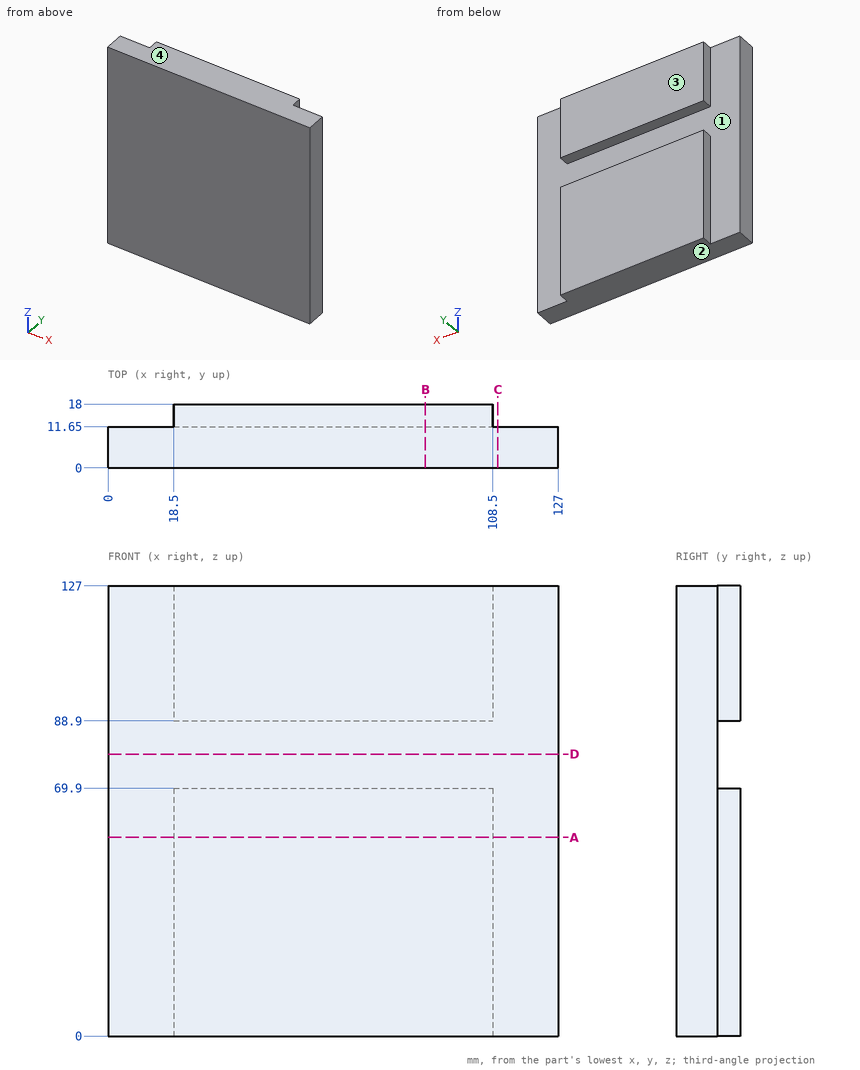
For this review, use the dimensioned drawing (mm, ordinates from the lowest corner) and the shaded views. Coordinates: 2 decimals unless noted, no trailing zeros. Loops run counter-clockwise (first coordinate to the right, second up) from the corner with the lowest first, then second, coordinate; pieces in that order, holes last. Notation, with made-up numbers: (9.25, -37) -> (47.25, -37) arc R27 cw to (47.25, -3) -> close; hole circle Ø1 at (52.5, 73). An arc over 180 degrees is marked (long way). Write each question's results on one line, items separated by ' | '.
Q1. Add section D-D, the plane z = 79.5. State the section outline as (x, y) points.
Taken from the geometry:
outline: (0, 0) -> (127, 0) -> (127, 11.65) -> (0, 11.65) -> close
Q2. To check wall thickness, follow line 1 along Z through (x, y) = (35.5, 14.25); line 2 along X through (y, z) = (12, 43.5); line 3 along Y through (x, z) = (26.5, 78). State the ranges of each line that lie inside material, in increasing order. Write a range as [from, to].
Taken from the geometry:
line 1: [0, 69.9], [88.9, 127] | line 2: [18.5, 108.5] | line 3: [0, 11.65]
Q3. Add section A-A, the plane z = 56. State the section outline as (x, y) points.
Taken from the geometry:
outline: (0, 0) -> (127, 0) -> (127, 11.65) -> (108.5, 11.65) -> (108.5, 18) -> (18.5, 18) -> (18.5, 11.65) -> (0, 11.65) -> close
Q4. Add section C-C, the plane x = 110. State the section outline as (y, z) points, then the cut area to 3 significant figures.
Taken from the geometry:
outline: (0, 0) -> (11.65, 0) -> (11.65, 127) -> (0, 127) -> close | area: 1,480 mm²
Q5. For pin 1 Ø3 at (y, z) = (14.5, 106) entering from +X; pin 2 Ø7 at (y, z) = (15.5, 45.5) entering from -X, all flat-tipped, find the tip position at first contact; note any pin that passes through.
Taken from the geometry:
pin 1: x = 108.5 | pin 2: x = 18.5
Q6. Add section B-B, the plane x = 89.5. State the section outline as (y, z) points.
Taken from the geometry:
outline: (0, 0) -> (18, 0) -> (18, 69.9) -> (11.65, 69.9) -> (11.65, 88.9) -> (18, 88.9) -> (18, 127) -> (0, 127) -> close
Q7. Mouldability with a two-part tool opening along Z and no side actions: class the marked faces 1, 2, 3 and 4 as +Z half, -Z half, draft (parallel to the pull), parting line (faces both ways), or undercut.
Taken from the geometry:
face 1: undercut | face 2: -Z half | face 3: draft | face 4: +Z half
